Input: part model. Units: mm. Frame: model coordinates. A direction names the side the tool comes from. Give positions to 0.01 mm unless a question says otherwise; leave off trailing zeros. Answer as a JSON object with one key per item and string values. Group by question number.
from build123d import *

# Parameters (mm, degrees)
F0_W     = 31.75
F0_H     = 666.75
F1_DEPTH = 31.75
F2_W     = 19.05
F2_H     = 6.35
F3_DEPTH = 25.4
F4_R     = 9.52499
F5_R     = 3.81
F6_DEPTH = 6.35
F7_W     = 1.5875
F7_H     = 12.7
F8_DEPTH = 22.225


# Not quite as in the source:
# - a fillet or chamfer is up to 0.001 mm smaller than in the source, because OpenCascade refuses the exact size


with BuildPart() as f1:
    # F0 (on Front) → F1 (new body)
    with BuildSketch(Plane.XZ):
        with Locations((-15.875, 127.5886728781)):
            Rectangle(F0_W, F0_H)
    extrude(amount=-F1_DEPTH)

    # F2 (on face) → F3 (join)
    with BuildSketch(Plane.XY.offset(460.9636728781)):
        with Locations((-15.875, 15.875)):
            Rectangle(F2_W, F2_H)
    extrude(amount=F3_DEPTH)

    # F4 (radius 9.525 in the source; OpenCascade refuses exactly that, so slightly less here)
    f4_edges = [f1.edges().sort_by_distance(p)[0] for p in [
        (-6.35, 15.875, 486.363673),
        (-25.4, 15.875, 486.363673),
    ]]
    fillet(f4_edges, radius=F4_R)

    # F5 (on face) → F6 (cut)
    with BuildSketch(Plane.XZ.offset(-12.7)):
        with Locations((-15.875, 476.8386728781)):
            Circle(F5_R)
    extrude(amount=-F6_DEPTH, mode=Mode.SUBTRACT)

    # F7 (on face) → F8 (cut)
    with BuildSketch(Plane(origin=(-31.75, 0, 0), x_dir=(0, -1, 0), z_dir=(-1, 0, 0))):
        with Locations((-29.36875, -177.2113271219)):
            Rectangle(F7_W, F7_H)
    extrude(amount=-F8_DEPTH, mode=Mode.SUBTRACT)


solid = f1.part
1. Line query: line 1 (Z direction, x = -5, y = 2). Output: solid intervals per line, ascending.
2. Reachability of faces 1 (the face through (-16, 0, 132)), 2 (the face through (-21, 28.575, -177)), 3 (the face through (-16, 12.7, 471)) from +Z, -Z, +X, -X, +Y, -Y: full face, straight path, thin tool, end or side. Return the list, or none.
3. Contact query for flat-ended pins moving along their axis: pin 1 Ø7 at (y, z) = (17, 469.5) entering from +X; pin 2 Ø1.5 at (y, z) = (9.5, 288.5) entering from +X; pin 3 Ø0.5 at (y, z) = (29.5, -180) entering from -X (3 decimals); pin 4 Ø1.7 at (x, y) = (-19, 29.5) entering from +Z. Output: stop coordinate, or through.
4. Mould query, pull axis Z, two halves, no side actions, for faces 4 (the face through (-21, 30.162, -177)), 5 (the face through (-16, 19.05, 471)), 6 (the face through (-16, 16, -205.786)). Classes: pulls with the +Z half, pulls with the -Z half, needs draft (parallel to the pull), parting line crosses it, or undercut.
Working result:
{
 "1": {"line 1": "z = -205.79 to 460.96"},
 "2": {"face 1": "+Z, -Z, +X, -X, -Y", "face 2": "-X", "face 3": "+Z, +X, -X, -Y"},
 "3": {"pin 1": "stops at x = -6.35", "pin 2": "stops at x = 0", "pin 3": "stops at x = -9.525", "pin 4": "stops at z = 460.96"},
 "4": {"face 4": "undercut", "face 5": "needs draft", "face 6": "pulls with the -Z half"}
}
